The model under review builds one solid part; all positions refer to its coordinate system, in mm. Face numbers are marked on the shaded views. A direction names the side the tool comes from. Round coordinates to 2 decimals unless told otherwise and drop trailing zeros. Order: outer loops, then holes, each group sorted by start corner. A loop starts at its lowest first (then second) coordinate and runs counter-clockwise, first axis right, second up.
1) Consider section A-A (y = 116). Give the boundary of the cut face in (x, z).
2) To check wall thickness, follow L1, parallel to Z at x = -104, y = 93.5; L2, parallel to Y at x = 127, z = -48.5; L3, parallel to Y at x = 118, z = -172. State the ranges of each line that lie inside material, in increasing order.
3) Machinability: for the marked faces 1 and 2, which of the approach directions +Z, -Z, +X, -X, +Y, -Y give a long, thin tool a straight path to every point of the face, cutting with its end or side? Answer none if there is none.
4) Consider section B-B (y = 91). Give the boundary of the cut face in (x, z), then the cut area to 3 significant figures.
5) Consider section C-C (x = -22). Give the boundary of the cut face in (y, z), then the cut area to 3 significant figures.
6) Mouldability with a two-part tool opening along Z and no side actions: class the marked faces 3, 4 and 5 as pulls with the +Z half, pulls with the -Z half, needs draft (parallel to the pull), parting line crosses it, or undercut.
7) Consider section D-D (z = -6). Give the boundary of the cut face in (x, y).
8) Clearance check with flat-ended pins moving along their axes: P1, Ø3.5, axis at x = -16.5, z = 172, coming from the +Y side; P2, Ø10, axis at x = 138.5, z = -16.5, coming from the +Y side; P3, Ø5.5, axis at x = -159.51, y = 124, coming from the -Z side. State where each tip first meets the part, or that it passes through.
from build123d import *

# Parameters (mm, degrees)
BASE_FLANGE1_DEPTH         = 3.302
SKETCHED_START             = -200.64222
SKETCHED_BEND1_DEPTH       = 401.28444
SKETCHED_BEND1_2_DEPTH     = 401.28444
SKETCHED_BEND1_3_OUTLINE_W = 25.4
SKETCHED_BEND1_3_OUTLINE_H = 3.302
SKETCHED_BEND1_3_DEPTH     = 124.44222
SKETCHED_START_2           = 76.2
SKETCHED_BEND1_4_OUTLINE_W = 25.4
SKETCHED_BEND1_4_OUTLINE_H = 3.302
SKETCHED_BEND1_4_DEPTH     = 124.44222
SKETCH15_R                 = 3.175
EXTRUDE2_DEPTH             = 424.025832199


# Read off the part's stored shape, not the designer's step: Sketched Bend1
# Sheet-metal steps are written as plain solids
with BuildPart() as part:
    # Sketch2 → Base-Flange1 (new body)
    with BuildSketch(Plane(origin=(0, 0, 0), x_dir=(1, 0, 0), z_dir=(0, 1, 0))):
        Polygon((200.64222, -301.9242367), (200.64222, 301.9242367), (76.2, 301.9242367), (76.2, 276.5242367), (-76.2, 276.5242367), (-76.2, 301.9242367), (-200.64222, 301.9242367), (-200.64222, -301.9242367), (-76.2, -301.9242367), (-76.2, -276.5242367), (76.2, -276.5242367), (76.2, -301.9242367), align=None)
    extrude(amount=BASE_FLANGE1_DEPTH)

    # Sketched Bend1 outline → Sketched Bend1 (cut)
    with BuildSketch(Plane.YZ.offset(SKETCHED_START)):
        with BuildLine():
            ThreePointArc((0, 167.224159597), (0.884768233, 170.526159597), (3.302, 172.943391364))
            Line((3.302, 172.943391364), (3.302, 301.9242367))
            Line((3.302, 301.9242367), (0, 301.9242367))
            Line((0, 301.9242367), (0, 167.224159597))
        make_face()
        with BuildLine():
            ThreePointArc((3.302, -172.943391364), (0.884768233, -170.526159597), (0, -167.224159597))
            Line((0, -167.224159597), (0, -301.9242367))
            Line((0, -301.9242367), (3.302, -301.9242367))
            Line((3.302, -301.9242367), (3.302, -172.943391364))
        make_face()
    extrude(amount=SKETCHED_BEND1_DEPTH, mode=Mode.SUBTRACT)

    # Sketched Bend1 2 outline → Sketched Bend1 2 (add)
    with BuildSketch(Plane.YZ.offset(SKETCHED_START)):
        with BuildLine():
            ThreePointArc((3.302, 167.224159597), (4.269133409, 169.559026188), (6.604, 170.526159597))
            Line((6.604, 170.526159597), (108.123922897, 170.526159597))
            Line((108.123922897, 170.526159597), (108.123922897, 173.828159597))
            Line((108.123922897, 173.828159597), (6.604, 173.828159597))
            ThreePointArc((6.604, 173.828159597), (4.894759026, 173.603133754), (3.302, 172.943391364))
            Line((3.302, 172.943391364), (3.302, 167.224159597))
        make_face()
        with BuildLine():
            ThreePointArc((6.604, -170.526159597), (4.269133409, -169.559026188), (3.302, -167.224159597))
            Line((3.302, -167.224159597), (3.302, -172.943391364))
            ThreePointArc((3.302, -172.943391364), (4.894759026, -173.603133754), (6.604, -173.828159597))
            Line((6.604, -173.828159597), (108.123922897, -173.828159597))
            Line((108.123922897, -173.828159597), (108.123922897, -170.526159597))
            Line((108.123922897, -170.526159597), (6.604, -170.526159597))
        make_face()
    extrude(amount=SKETCHED_BEND1_2_DEPTH)

    # Sketched Bend1 3 outline → Sketched Bend1 3 (add)
    with BuildSketch(Plane.YZ.offset(SKETCHED_START)):
        with Locations((120.823922897, 172.177159597)):
            Rectangle(SKETCHED_BEND1_3_OUTLINE_W, SKETCHED_BEND1_3_OUTLINE_H)
        with Locations((120.823922897, -172.177159597)):
            Rectangle(SKETCHED_BEND1_3_OUTLINE_W, SKETCHED_BEND1_3_OUTLINE_H)
    extrude(amount=SKETCHED_BEND1_3_DEPTH)

    # Sketched Bend1 4 outline → Sketched Bend1 4 (add)
    with BuildSketch(Plane.YZ.offset(SKETCHED_START_2)):
        with Locations((120.823922897, 172.177159597)):
            Rectangle(SKETCHED_BEND1_4_OUTLINE_W, SKETCHED_BEND1_4_OUTLINE_H)
        with Locations((120.823922897, -172.177159597)):
            Rectangle(SKETCHED_BEND1_4_OUTLINE_W, SKETCHED_BEND1_4_OUTLINE_H)
    extrude(amount=SKETCHED_BEND1_4_DEPTH)

    # Sketch15 → Extrude2 (cut, through all)
    with BuildSketch(Plane.XY.offset(173.828159597)):
        with Locations((-159.512, 123.998922897)):
            Circle(SKETCH15_R)
        with Locations((-118.11, 123.998922897)):
            Circle(SKETCH15_R)
        with Locations(Location((118.11, 123.998922897, 0), (0, 0, 270))):
            Circle(SKETCH15_R)
        with Locations(Location((159.512, 123.998922897, 0), (0, 0, 270))):
            Circle(SKETCH15_R)
    extrude(amount=-EXTRUDE2_DEPTH, mode=Mode.SUBTRACT)


solid = part.part
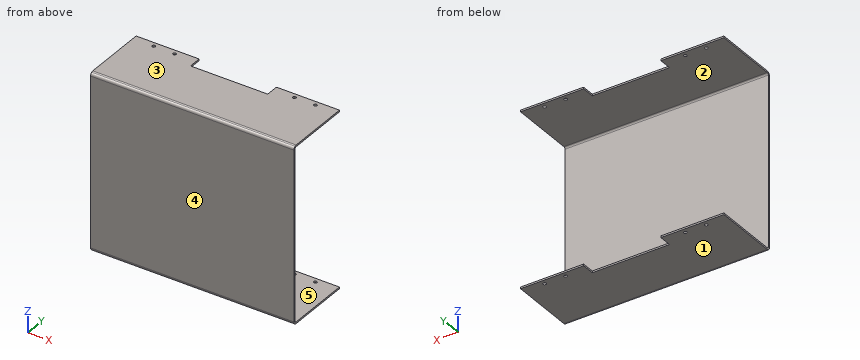
Answer below:
1. outline: (-200.64, -173.83) - (-76.2, -173.83) - (-76.2, -170.53) - (-200.64, -170.53) - close; (-200.64, 170.53) - (-76.2, 170.53) - (-76.2, 173.83) - (-200.64, 173.83) - close; (76.2, -173.83) - (200.64, -173.83) - (200.64, -170.53) - (76.2, -170.53) - close; (76.2, 170.53) - (200.64, 170.53) - (200.64, 173.83) - (76.2, 173.83) - close
2. L1: z = -173.83 to -170.53, 170.53 to 173.83
2. L2: y = 0 to 3.3
2. L3: y = 2.04 to 120.83, 127.17 to 133.52
3. face 1: -Z, +X, -X, +Y, -Y
3. face 2: +X, -X, +Y
4. outline: (-200.64, -173.83) - (200.64, -173.83) - (200.64, -170.53) - (-200.64, -170.53) - close; (-200.64, 170.53) - (200.64, 170.53) - (200.64, 173.83) - (-200.64, 173.83) - close
4. area: 2,650 mm2
5. outline: (0, -167.22) arc R6.6 ccw to (6.6, -173.83) - (108.12, -173.83) - (108.12, -170.53) - (6.6, -170.53) arc R3.3 cw to (3.3, -167.22) - (3.3, 167.22) arc R3.3 cw to (6.6, 170.53) - (108.12, 170.53) - (108.12, 173.83) - (6.6, 173.83) arc R6.6 ccw to (0, 167.22) - close
5. area: 1,830 mm2
6. face 3: pulls with the +Z half
6. face 4: needs draft
6. face 5: undercut
7. outline: (-200.64, 0) - (200.64, 0) - (200.64, 3.3) - (-200.64, 3.3) - close
8. P1: stops at y = 108.12
8. P2: stops at y = 3.3
8. P3: passes through
